Answer from the drawing. Dimensions are ordinates in mm from the lowest x, y and z of the part. A direction names the side the tool comes from. Round coordinates to 2 decimals unless told otherwise and drop trailing zeros. Write each loop counter-clockwise with the first axis right and the second up, starting at its lowest first coordinate (ties: lowest second). Pieces come first, ordered by that corner, then holes. Notation, with made-up numbers: (64.25, 80) - (88.25, 80) arc R31 ccw to (88.25, 104) - close; hole circle Ø3 at (-26.75, 46.5). An arc over 180 degrees is marked (long way). Answer as a JSON object with one key per item and string values.
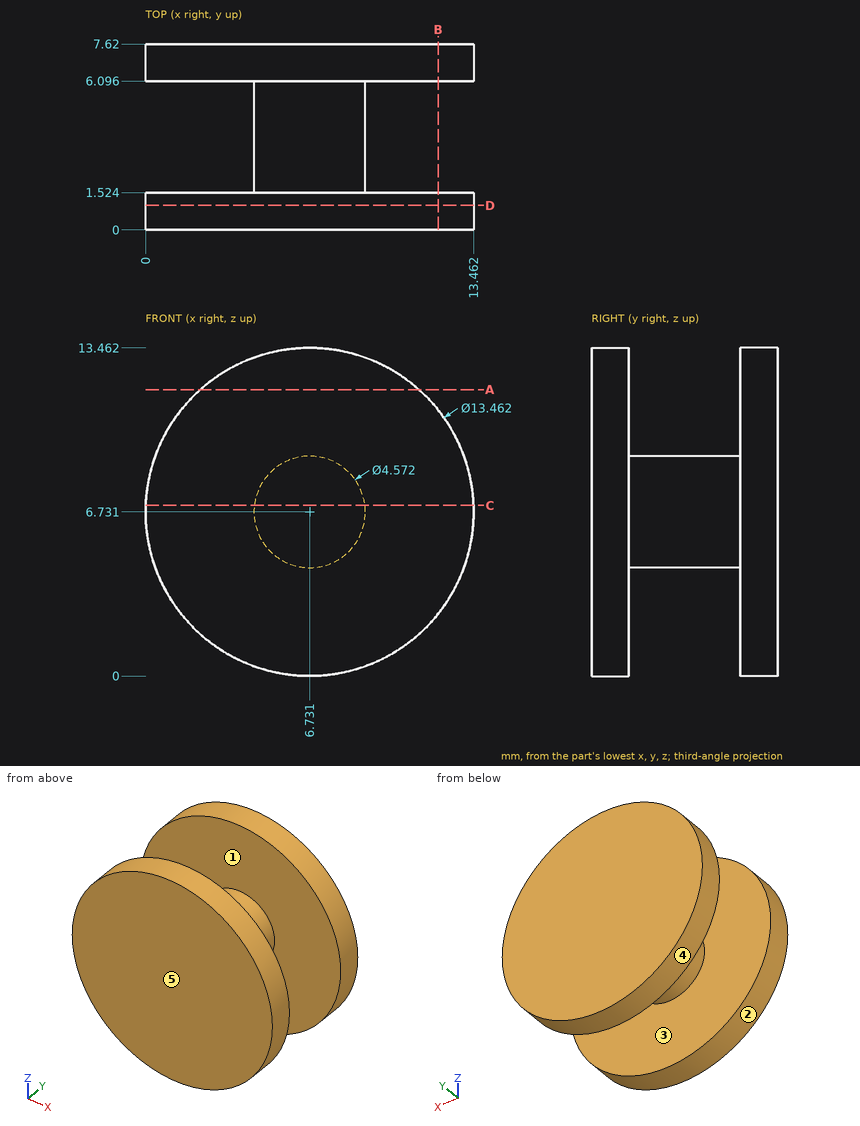
Item 1: A cutting plane is placed at A-A (z = 11.75). Write down the section's boundary in (x, y).
Results found:
{"outline": "(2.25, 0) - (11.22, 0) - (11.22, 1.52) - (2.25, 1.52) - close; (2.25, 6.1) - (11.22, 6.1) - (11.22, 7.62) - (2.25, 7.62) - close"}
Item 2: For the marked faces 1 and 2, determine the directions among +Z, -Z, +X, -X, +Y, -Y from which every point of the face is accessible in a straight line to the end or side of a thin tool.
Results found:
{"face 1": "none", "face 2": "+Y, -Y"}
Item 3: A cutting plane is placed at B-B (x = 12). Write down the section's boundary in (y, z), and give its area (3 significant figures).
Results found:
{"outline": "(0, 2.54) - (1.52, 2.54) - (1.52, 10.92) - (0, 10.92) - close; (6.1, 2.54) - (7.62, 2.54) - (7.62, 10.92) - (6.1, 10.92) - close", "area": "25.5 mm²"}
Item 4: A cutting plane is placed at C-C (z = 7). Write down the section's boundary in (x, y), and give its area (3 significant figures).
Results found:
{"outline": "(0.01, 0) - (13.46, 0) - (13.46, 1.52) - (9, 1.52) - (9, 6.1) - (13.46, 6.1) - (13.46, 7.62) - (0.01, 7.62) - (0.01, 6.1) - (4.46, 6.1) - (4.46, 1.52) - (0.01, 1.52) - close", "area": "61.8 mm²"}
Item 5: Consider line 1 along Y through (x, z) = (4.5, 3.25); line 2 along X through (y, z) = (7.5, 4.75); line 3 along Z through (x, y) = (8, 6.75). Determine where each line is inside the solid, lowest interval first.
Results found:
{"line 1": "0 to 1.52, 6.1 to 7.62", "line 2": "0.3 to 13.16", "line 3": "0.12 to 13.34"}
Item 6: Each of these flat-tipped pins is pushed along its axis until it touches: P1, Ø3, axis at x = 4.5, y = 5, coming from the -Z side; P2, Ø2, axis at y = 5.5, z = 5.5, coming from the -X side; P3, Ø1, axis at y = 3, z = 5.5, coming from the +X side. Where does it stop, or does it pass through?
Results found:
{"P1": "z = 0.11", "P2": "x = 0.01", "P3": "x = 8.9"}
Item 7: A cutting plane is placed at D-D (y = 1). Write down the section's boundary in (x, z), and give its area (3 significant figures).
Results found:
{"outline": "circle Ø13.46 at (6.73, 6.73)", "area": "142 mm²"}
Item 8: Determine the mould class of the marked faces 3, 4 and 5 for opening direction Y: pulls with the +Y half, pulls with the -Y half, needs draft (parallel to the pull), parting line crosses it, or undercut.
Results found:
{"face 3": "undercut", "face 4": "needs draft", "face 5": "pulls with the -Y half"}
